Autodesk Inventor part; units mm, degrees
ref_plane "YZ Plane" through (0, 0, 0) normal (1, 0, 0) x (0, 1, 0)
ref_plane "XZ Plane" through (0, 0, 0) normal (0, 1, 0) x (-1, 0, 0)
ref_plane "XY Plane" through (0, 0, 0) normal (0, 0, 1) x (1, 0, 0)
sketch "Sketch1" plane through (0, 0, 0) normal (0, 0, 1) x (1, 0, 0)
  line L0 (-26, 12.85) -> (26, 12.85)
  line L1 (26, 12.85) -> (26, 6.85)
  line L2 (5, -7.15) -> (-5, -7.15)
  line L3 (-26, 6.85) -> (-26, 12.85)
  line L4 (-22, -5.35) -> (-22, 5.35)
  line L5 (22, -5.35) -> (22, 5.35)
  line L6 (-22, 6.85) -> (-26, 6.85)
  line L7 (22, 6.85) -> (26, 6.85)
  line L8 (0, 5.6029) -> (0, -5.6029) construction
  arc A0 (-22, 5.35) -> (-22, 6.85) centre (-22, 6.1) ccw
  arc A1 (22, 6.85) -> (22, 5.35) centre (22, 6.1) ccw
  line L9 (-5, -7.15) -> (-5, -5.35)
  line L10 (-6.5, -5.35) -> (-22, -5.35)
  line L11 (5, -7.15) -> (5, -5.35)
  line L12 (6.5, -5.35) -> (22, -5.35)
  arc A2 (-5, -5.35) -> (-6.5, -5.35) centre (-5.75, -5.35) ccw
  arc A3 (6.5, -5.35) -> (5, -5.35) centre (5.75, -5.35) ccw
  point P0 (0, 0)
  point P1 (0, 12.85)
  point P2 (26, 0)
  point P3 (0, 0)
  point P4 (-22, 0)
  dimension "d0" = 52
  dimension "d4" = 44
  dimension "d6" = 20
  dimension "d7" = 6
  dimension "d8" = 1.5
  dimension "d18" = 10
  dimension "d19" = 1.8
  dimension "d20" = 1.5
extrude "Extrusion1" add sketch "Sketch1" along normal blind 1.6
sketch "Sketch2" plane through (0, 0, 1.6) normal (0, 0, 1) x (1, 0, 0)
  point P0 (0, 0)
  point P1 (-15, 2.97)
  point P2 (0, 2.97)
  point P3 (15, 2.97)
  dimension "d9" = 15
  dimension "d10" = 15
properties part number "AK-C-C10-Insert-Board"
Design review of the part built by this model. Coordinates are the model's own, in mm. A direction names the side the tool comes from. Round coordinates to 2 decimals unless told otherwise and drop trailing zeros. Write each loop counter-clockwise with the first axis right and the second up, starting at its lowest first coordinate (ties: lowest second). Pieces come first, ordered by that corner, then holes. Notation, with made-up numbers: (59.25, 42) - (101.25, 42) arc R18 ccw to (101.25, 55) - close; hole circle Ø4 at (87.5, -20). An arc over 180 degrees is marked (long way). Use a Markdown table: item, result. Add a question column.
1. Clearance check with flat-ended pins moving along their axes: pin 1 (0.8 mm diameter, centred on y = 1.5, z = 0.5, fed in from +X); pin 2 (0.5 mm diameter, centred on x = 16.5, z = 1, fed in from -Y); pin 3 (0.5 mm diameter, centred on y = 0.5, z = 0.5, fed in from -X). State where each tip first meets the part, or that it passes through.
2. We need section C-C (y = 0). State the section outline as (x, z) points, then the cut area to 3 significant figures.
3. Wall thickness on probe 1 along X at (y, z) = (-5, 1.05); probe 2 along Y at (x, z) = (-8, 0.5); probe 3 along X at (y, z) = (-6, 0.4): over which ranges is each line inside the solid? List them lowest first.
4. Mouldability with a two-part tool opening along Y and no side actions: class faces 1 (the face through (-21.25, 6.12, 0.79)), 2 (the face through (0, 12.85, 1)), 3 (the face through (5.7, -4.6, 0.8)), 4 (the face through (-22, 0, 1)) as +Y half, -Y half, draft (parallel to the pull), parting line (faces both ways), or undercut.
5. For faces 5 (the face through (21.25, 6.08, 0.79)), 6 (the face through (22, 0, 1)), 7 (the face through (-5, -6, 1)), list the 3-axis set-ups (+Z, -Z, +X, -X, +Y, -Y) from which the entire face can be reached by the end or side of a thin tool; tool diameter is ignored.
6. We need section B-B (x = -5.75). State the section outline as (y, z) points, then the cut area to 3 significant figures.
7. We need section A-A (z = 0.7). State the section outline as (x, y) points.
Output:
| question | item | result |
|---|---|---|
| 1 | pin 1 | stops at x = 22 |
| 1 | pin 2 | stops at y = -5.35 |
| 1 | pin 3 | stops at x = -22 |
| 2 | outline | (-22, 0) - (22, 0) - (22, 1.6) - (-22, 1.6) - close |
| 2 | area | 70.4 mm2 |
| 3 | probe 1 | x = -22 to -6.41, -5.09 to 5.09, 6.41 to 22 |
| 3 | probe 2 | y = -5.35 to 12.85 |
| 3 | probe 3 | x = -5 to 5 |
| 4 | face 1 | undercut |
| 4 | face 2 | +Y half |
| 4 | face 3 | -Y half |
| 4 | face 4 | draft |
| 5 | face 5 | +Z, -Z, +X |
| 5 | face 6 | +Z, -Z, +X, -Y |
| 5 | face 7 | +Z, -Z, -X, -Y |
| 6 | outline | (-4.6, 0) - (12.85, 0) - (12.85, 1.6) - (-4.6, 1.6) - close |
| 6 | area | 27.9 mm2 |
| 7 | outline | (-26, 6.85) - (-22, 6.85) arc R0.75 cw to (-22, 5.35) - (-22, -5.35) - (-6.5, -5.35) arc R0.75 cw to (-5, -5.35) - (-5, -7.15) - (5, -7.15) - (5, -5.35) arc R0.75 cw to (6.5, -5.35) - (22, -5.35) - (22, 5.35) arc R0.75 cw to (22, 6.85) - (26, 6.85) - (26, 12.85) - (-26, 12.85) - close |
